from build123d import *

# Parameters (mm, degrees)
CROQUIS1_W              = 600
CROQUIS1_H              = 600
CROQUIS1_R              = 187.5
SALIENTE_EXTRUIR1_DEPTH = 120
CROQUIS3_W              = 80
CROQUIS3_H              = 90
CORTAR_EXTRUIR2_DEPTH   = 80
CROQUIS5_W              = 80
CROQUIS5_H              = 90
CORTAR_EXTRUIR3_DEPTH   = 90
CORTAR_EXTRUIR4_DEPTH   = 80
CROQUIS7_W              = 89.245379234
CROQUIS7_H              = 80
CORTAR_EXTRUIR5_DEPTH   = 90
CORTAR_EXTRUIR13_DEPTH  = 80
CROQUIS10_W             = 90
CROQUIS10_H             = 80
CORTAR_EXTRUIR15_DEPTH  = 90
CORTAR_EXTRUIR17_DEPTH  = 80
CROQUIS12_W             = 80
CROQUIS12_H             = 90
CORTAR_EXTRUIR19_DEPTH  = 90
CROQUIS13_R             = 80
CORTAR_EXTRUIR20_DEPTH  = 10
CROQUIS14_R             = 80
CORTAR_EXTRUIR21_DEPTH  = 10


with BuildPart() as part:
    # Croquis1 → Saliente-Extruir1 (new body)
    with BuildSketch(Plane.XY):
        Rectangle(CROQUIS1_W, CROQUIS1_H)
        Circle(CROQUIS1_R, mode=Mode.SUBTRACT)
    extrude(amount=SALIENTE_EXTRUIR1_DEPTH)

    # Croquis3 → Cortar-Extruir2 (cut)
    with BuildSketch(Plane.ZY.offset(300)):
        Polygon((0, 210), (0, -210), (80, -210), align=None)
        with Locations((40, 255)):
            Rectangle(CROQUIS3_W, CROQUIS3_H)
    extrude(amount=-CORTAR_EXTRUIR2_DEPTH, mode=Mode.SUBTRACT)

    # Croquis5 → Cortar-Extruir3 (cut)
    with BuildSketch(Plane.ZY.offset(300)):
        with Locations((40, -255)):
            Rectangle(CROQUIS5_W, CROQUIS5_H)
    extrude(amount=-CORTAR_EXTRUIR3_DEPTH, mode=Mode.SUBTRACT)

    # Croquis6 → Cortar-Extruir4 (cut)
    with BuildSketch(Plane(origin=(0, 300, 0), x_dir=(1, 0, 0), z_dir=(0, 1, 0))):
        Polygon((-210, -80), (210, 0), (-210, 0), align=None)
    extrude(amount=-CORTAR_EXTRUIR4_DEPTH, mode=Mode.SUBTRACT)

    # Croquis7 → Cortar-Extruir5 (cut)
    with BuildSketch(Plane(origin=(0, 300, 0), x_dir=(1, 0, 0), z_dir=(0, 1, 0))):
        with Locations((-254.622689617, -40)):
            Rectangle(CROQUIS7_W, CROQUIS7_H)
    extrude(amount=-CORTAR_EXTRUIR5_DEPTH, mode=Mode.SUBTRACT)

    # Croquis8 → Cortar-Extruir13 (cut)
    with BuildSketch(Plane(origin=(300, 0, 0), x_dir=(0, 0, -1), z_dir=(1, 0, 0))):
        Polygon((-80, 210), (0, -210), (0, 210), align=None)
    extrude(amount=-CORTAR_EXTRUIR13_DEPTH, mode=Mode.SUBTRACT)

    # Croquis10 → Cortar-Extruir15 (cut)
    with BuildSketch(Plane(origin=(0, 300, 0), x_dir=(1, 0, 0), z_dir=(0, 1, 0))):
        with Locations((255, -40)):
            Rectangle(CROQUIS10_W, CROQUIS10_H)
    extrude(amount=-CORTAR_EXTRUIR15_DEPTH, mode=Mode.SUBTRACT)

    # Croquis11 → Cortar-Extruir17 (cut)
    with BuildSketch(Plane.XZ.offset(300)):
        Polygon((210, 80), (-210, 0), (210, 0), align=None)
    extrude(amount=-CORTAR_EXTRUIR17_DEPTH, mode=Mode.SUBTRACT)

    # Croquis12 → Cortar-Extruir19 (cut)
    with BuildSketch(Plane(origin=(300, 0, 0), x_dir=(0, 0, -1), z_dir=(1, 0, 0))):
        with Locations((-40, -255)):
            Rectangle(CROQUIS12_W, CROQUIS12_H)
    extrude(amount=-CORTAR_EXTRUIR19_DEPTH, mode=Mode.SUBTRACT)

    # Croquis13 → Cortar-Extruir20 (cut)
    with BuildSketch(Plane.XY.offset(120)):
        with Locations((-200, 200)):
            Circle(CROQUIS13_R)
    extrude(amount=-CORTAR_EXTRUIR20_DEPTH, mode=Mode.SUBTRACT)

    # Croquis14 → Cortar-Extruir21 (cut)
    with BuildSketch(Plane.XY.offset(120)):
        with Locations((-210, -210)):
            Circle(CROQUIS14_R)
        with Locations((210, -210)):
            Circle(CROQUIS14_R)
        with Locations((210, 210)):
            Circle(CROQUIS14_R)
    extrude(amount=-CORTAR_EXTRUIR21_DEPTH, mode=Mode.SUBTRACT)


solid = part.part
Check sheet for the modelled part. Datum: model origin and axes. Units: mm. A direction names the side the tool comes from. Round coordinates to 2 decimals unless told otherwise and drop trailing zeros. Write each loop counter-clockwise with the first axis right and the second up, starting at its lowest first coordinate (ties: lowest second). Pieces come first, ordered by that corner, then holes. Notation, with made-up numbers: (77, -7.5) -> (103, -7.5) arc R26 cw to (103, 19.5) -> close; hole circle Ø10 at (87.5, -5.75). An arc over 180 degrees is marked (long way). Answer as CSV lines item,"result". Start each with the question number.
1) Section check B-B on x = 0. Enter the section's corners in (y, z).
2) Section check D-D on z = 22. Enter the section's corners in (x, y), and give its area (3 significant figures).
3) Go/stop test with flat-tipped pins: P1, Ø8, axis at y = 213.5, z = 57, coming from the -X side; P2, Ø3, axis at y = -215.5, z = 56.5, coming from the +X side; P3, Ø6, axis at y = 133, z = 34.5, coming from the +X side; P4, Ø2, axis at x = -153, y = -166.5, coming from the +Z side. Record where each tip stops, or that it passes through.
4) Tool access check on faces 1 (the flat face through (-201, 201, 110)), 2 (the flat face through (-2.94, 260.56, 40.56)), 3 (the flat face through (256, -256, 80)), 4 (the flat face through (-220, -90, 22)), 5 (the flat face through (220, 96, 23)). Record the directions out of +Z, -Z, +X, -X, +Y, -Y that give a thin tool (end or side, any length) a straight path to the whole face; none if there is none.
5) Section check A-A on z = 58. Enter the section's corners in (x, y), and give its area (3 significant figures).
6) Material ranges on line 1 (Y direction, x = 210, z = 117.75); line 2 (Y direction, x = -210, z = 114.5); line 3 (X direction, y = 86.5, z = 18.5), recorded low to high. Write a range as from..to.
7) Release check for a two-part mould opening along Y. For faces 6 (the cylindrical face through (100.8, 158.1, 59.2)), 7 (the flat face through (-50, 220, 31)), 8 (the flat face through (256, -210, 41)), 9 (the flat face through (-210, -254, 39)) record: pulls with the +Y half, pulls with the -Y half, needs draft (parallel to the pull), parting line crosses it, or undercut.
Found:
1,outline,"(-300, 40) -> (-220, 40) -> (-220, 0) -> (-187.5, 0) -> (-187.5, 120) -> (-300, 120) -> close; (187.5, 0) -> (220, 0) -> (220, 40) -> (300, 40) -> (300, 120) -> (187.5, 120) -> close"
2,outline,"(-300, 94.5) -> (-220, 94.5) -> (-220, -210) -> (-210, -210) -> (-210, -300) -> (-94.5, -300) -> (-94.5, -220) -> (210, -220) -> (210, -210) -> (300, -210) -> (300, -94.5) -> (220, -94.5) -> (220, 210) -> (210, 210) -> (210, 300) -> (94.5, 300) -> (94.5, 220) -> (-210, 220) -> (-210, 210) -> (-300, 210) -> close; hole circle Ø375 at (0, 0)"
2,area,"120,000 mm^2"
3,P1,"stops at x = -300"
3,P2,"stops at x = 210"
3,P3,"stops at x = 220"
3,P4,"stops at z = 110"
4,face 1,"+Z"
4,face 2,"-Z, -X, +Y"
4,face 3,"-Z, +X, -Y"
4,face 4,"-Z, -X, -Y"
4,face 5,"-Z, +X, +Y"
5,outline,"(-300, -94.5) -> (-220, -94.5) -> (-220, -210) -> (-210, -210) -> (-210, -300) -> (94.5, -300) -> (94.5, -220) -> (210, -220) -> (210, -210) -> (300, -210) -> (300, 94.5) -> (220, 94.5) -> (220, 210) -> (210, 210) -> (210, 300) -> (-94.5, 300) -> (-94.5, 220) -> (-210, 220) -> (-210, 210) -> (-300, 210) -> close; hole circle Ø375 at (0, 0)"
5,area,"180,000 mm^2"
6,line 1,"y = -300..-290, -130..130, 290..300"
6,line 2,"y = -300..-290, -130..120.63, 279.37..300"
6,line 3,"x = -220..-166.36, 166.36..220"
7,face 6,"undercut"
7,face 7,"pulls with the +Y half"
7,face 8,"pulls with the -Y half"
7,face 9,"needs draft"
